Design review of the part built by this model. Coordinates are the model's own, in mm. A direction names the side the tool comes from. Coordinates: 2 decimals unless noted, no trailing zeros. Loops run counter-clockwise (first coordinate to the right, second up) from the corner with the lowest first, then second, coordinate; pieces in that order, holes last. Notation, with made-up numbers: (-12.75, 87.25) -> (23.25, 87.25) arc R30 cw to (23.25, 119.25) -> close; hole circle Ø9 at (78.25, 40.25). An arc over 180 degrees is marked (long way). One line per item, written item: value. Start each with the question number.
1. Add section C-C on x = 0. Write out the cut boundary in (y, z) (1 decimal), plus the area to 3 significant figures.
2. Machinability: for faces 5 (the cylindrical face through (-11.19, 0.49, 22.7)), 6 (the cylindrical face through (-11.78, -20.32, 22.7)), which of the approach directions +Z, -Z, +X, -X, +Y, -Y give a long, thin tool a straight path to every point of the face, cutting with its end or side? Answer none if there is none.
3. Add section A-A on x = 12.5. Write out the cut boundary in (y, z) (1 decimal), plus the area to 3 significant figures.
4. Insertion check: pin 1 (4 mm diameter, centred on y = -24.5, z = 20.5, fed in from +X); pin 2 (10 mm diameter, centred on y = 19, z = 40, fed in from +X); pin 3 (22 mm diameter, centred on y = -2.5, z = 22.5, fed in from +X) (3 decimals); pin 4 (3 mm diameter, centred on x = 16, y = 27.5, fed in from -Z). Each pin has a flat end and moves straight along its axis. Give the tip position at first contact, or say it passes through.
5. For probe 1 along Y at (x, z) = (0, 10) (3 decimals); probe 2 along Y at (x, z) = (13.5, 2) (3 decimals); probe 3 along Y at (x, z) = (-7, 32.5) (3 decimals), list the stretches that pass through material, from the lowest coordinate up.
6. Add section B-B on y = 0. Write out the cut boundary in (x, z) (1 decimal).
7. Draft analysis for pull direction Y (two halves, no side actions). For faces 1 (the flat face through (2, -19.455, 23)), 2 (the cylindrical face through (-11.783, 28.511, 22.696)), 3 (the flat face through (6, 42.08, 23)), 4 (the flat face through (7, -73.83, 23)), state which applies: pulls with the +Y half, pulls with the -Y half, needs draft (parallel to the pull), parting line crosses it, or undercut.
```python
from build123d import *

# Parameters (mm, degrees)
SKETCH1_R           = 11.2
BOSS_EXTRUDE1_DEPTH = 46.0375


with BuildPart() as part:
    # Sketch1 → Boss-Extrude1 (new body)
    with BuildSketch(Plane.XY):
        with BuildLine():
            Line((-25.4, -67.479999962), (-25.4, 36.365))
            ThreePointArc((-25.4, 36.365), (-23.726115254, 40.406115254), (-19.685, 42.08))
            Line((-19.685, 42.08), (32.385, 42.08))
            ThreePointArc((32.385, 42.08), (36.426115254, 40.406115254), (38.1, 36.365))
            Line((38.1, 36.365), (38.1, 35.095))
            ThreePointArc((38.1, 35.095), (36.426115254, 31.053884746), (32.385, 29.38))
            Line((32.385, 29.38), (-9.652, 29.38))
            ThreePointArc((-9.652, 29.38), (-11.807261469, 28.487261469), (-12.7, 26.332))
            Line((-12.7, 26.332), (-12.7, 22.503))
            ThreePointArc((-12.7, 22.503), (-11.807261469, 20.347738531), (-9.652, 19.455))
            Line((-9.652, 19.455), (0, 19.455))
            Line((0, 19.455), (13.74, 19.455))
            ThreePointArc((13.74, 19.455), (17.781115254, 17.781115254), (19.455, 13.74))
            Line((19.455, 13.74), (19.455, 0))
            Line((19.455, 0), (19.455, -13.74))
            ThreePointArc((19.455, -13.74), (17.781115254, -17.781115254), (13.74, -19.455))
            Line((13.74, -19.455), (0, -19.455))
            Line((0, -19.455), (-9.652, -19.455))
            ThreePointArc((-9.652, -19.455), (-11.807261469, -20.347738531), (-12.7, -22.503))
            Line((-12.7, -22.503), (-12.7, -26.331999962))
            ThreePointArc((-12.7, -26.331999962), (-11.807261469, -28.487261431), (-9.652, -29.379999962))
            Line((-9.652, -29.379999962), (32.385, -29.379999962))
            ThreePointArc((32.385, -29.379999962), (36.426115254, -31.053884708), (38.1, -35.094999962))
            Line((38.1, -35.094999962), (38.1, -67.479999962))
            ThreePointArc((38.1, -67.479999962), (36.240128061, -71.970128023), (31.75, -73.829999962))
            Line((31.75, -73.829999962), (-19.05, -73.829999962))
            ThreePointArc((-19.05, -73.829999962), (-23.540128061, -71.970128023), (-25.4, -67.479999962))
        make_face()
        Circle(SKETCH1_R, mode=Mode.SUBTRACT)
    extrude(amount=BOSS_EXTRUDE1_DEPTH)


solid = part.part
```
Worked answers:
1. outline: (-73.8, 0) -> (-29.4, 0) -> (-29.4, 46) -> (-73.8, 46) -> close; (-19.5, 0) -> (-11.2, 0) -> (-11.2, 46) -> (-19.5, 46) -> close; (11.2, 0) -> (19.5, 0) -> (19.5, 46) -> (11.2, 46) -> close; (29.4, 0) -> (42.1, 0) -> (42.1, 46) -> (29.4, 46) -> close
1. area: 3,390 mm²
2. face 5: +Z, -Z
2. face 6: +Z, -Z, +X
3. outline: (-73.8, 0) -> (-29.4, 0) -> (-29.4, 46) -> (-73.8, 46) -> close; (-19.5, 0) -> (19.5, 0) -> (19.5, 46) -> (-19.5, 46) -> close; (29.4, 0) -> (42.1, 0) -> (42.1, 46) -> (29.4, 46) -> close
3. area: 4,420 mm²
4. pin 1: stops at x = -12.7
4. pin 2: stops at x = 19.45
4. pin 3: stops at x = 19.455
4. pin 4: passes through
5. probe 1: y = -73.83 to -29.38, -19.455 to -11.2, 11.2 to 19.455, 29.38 to 42.08
5. probe 2: y = -73.83 to -29.38, -19.455 to 19.455, 29.38 to 42.08
5. probe 3: y = -73.83 to -29.38, -19.455 to -8.743, 8.743 to 19.455, 29.38 to 42.08
6. outline: (-25.4, 0) -> (-11.2, 0) -> (-11.2, 46) -> (-25.4, 46) -> close; (11.2, 0) -> (19.5, 0) -> (19.5, 46) -> (11.2, 46) -> close
7. face 1: undercut
7. face 2: undercut
7. face 3: pulls with the +Y half
7. face 4: pulls with the -Y half
